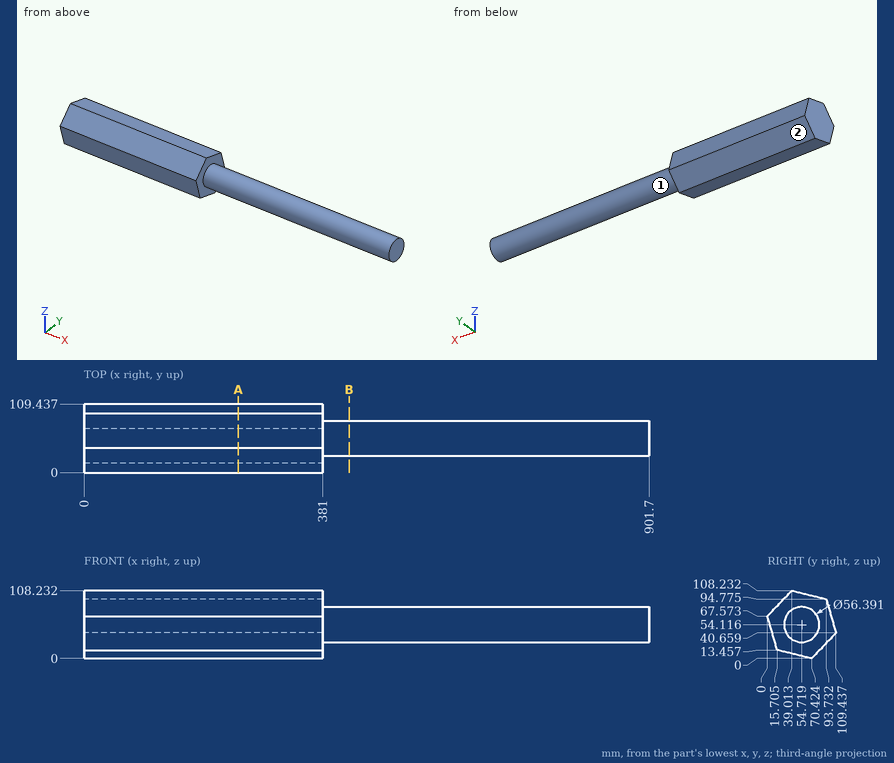
The drawing under review shows one solid part. Ordinate dimensions are in mm from its lowest x, y, z. A direction names the side the tool comes from. Give positions to 0.01 mm unless a question says otherwise; leave off trailing zeros. Order: outer loops, then holes, each group sorted by start corner. A loop starts at its lowest first (then second) coordinate and runs counter-clockwise, first axis right, second up. Notation, with made-up numbers: (24, 62) -> (71, 62) arc R13 cw to (71, 84) -> close; hole circle Ø2 at (38, 58.25). An arc over 180 degrees is marked (long way). Write item = value, one per line. Start each with the question number.
(1) We need section B-B on x = 423. Write out the cut boundary in (y, z) (1 decimal).
(2) To check wall thickness, follow line 1 along X through (y, z) = (34.5, 12); line 2 along Y through (x, z) = (747, 57); line 3 along Y through (x, z) = (108, 21) (1 decimal). State the ranges of each line that lie inside material, in increasing order.
(3) We need section A-A on x = 246. Write out the cut boundary in (y, z) (1 decimal), plus the area to 3 significant figures.
(4) For the marked faces 1 and 2, list the 3-axis set-ups (+Z, -Z, +X, -X, +Y, -Y) from which the entire face can be reached by the end or side of a thin tool; tool diameter is ignored.
(5) For pin 1 (8 mm diameter, centred on y = 46, z = 27, fed in from -X); pin 2 (3 mm diameter, centred on x = 405.5, y = 79, fed in from -Z) (1 decimal); pin 3 (2 mm diameter, centred on x = 734.5, y = 78, fed in from +Z) (1 decimal); pin 4 (12 mm diameter, centred on y = 88.5, z = 79.5, fed in from +X), all flat-tipped, find the tip position at first contact; note any pin that passes through.
Numbers:
q1.outline = circle Ø56.4 at (54.7, 54.1)
q2.line_1 = 0 to 381
q2.line_2 = 26.67 to 82.77
q2.line_3 = 13.5 to 90.6
q3.outline = (0, 67.6) -> (15.7, 13.5) -> (70.4, 0) -> (109.4, 40.7) -> (93.7, 94.8) -> (39, 108.2) -> close
q3.area = 8,250 mm^2
q4.face_1 = +X
q4.face_2 = -Z, +X, -X, +Y
q5.pin_1 = 0
q5.pin_2 = 37.5
q5.pin_3 = 71.4
q5.pin_4 = 381
